Source: three-view drawing plus pictorial views. Frame: mm from the lowest corner of the part. Give positions to 0.01 mm unless a question says otherwise; leave off trailing zeros. Write each loop counter-clockwise with the first axis right and the second up, starting at its lowest first coordinate (ties: lowest second). Pieces come first, ordered by that corner, then holes.
Q1. Cut plane A-A on z = 32. Return the cut outline in (x, y).
Q2. Line query: L1, parallel to X at y = 2.05, z = 3.5; L2, parallel to X at y = 2.55, z = 32; L3, parallel to Z at x = 79.5, y = 2. Output: solid intervals per line, ascending.
Q3. Cut plane B-B on x = 79.5. Return the cut outline in (y, z), plus the area to 3 significant figures.
Q4. Cut plane C-C on z = 3.5. Return the cut outline in (x, y), plus the area to 3 significant figures.
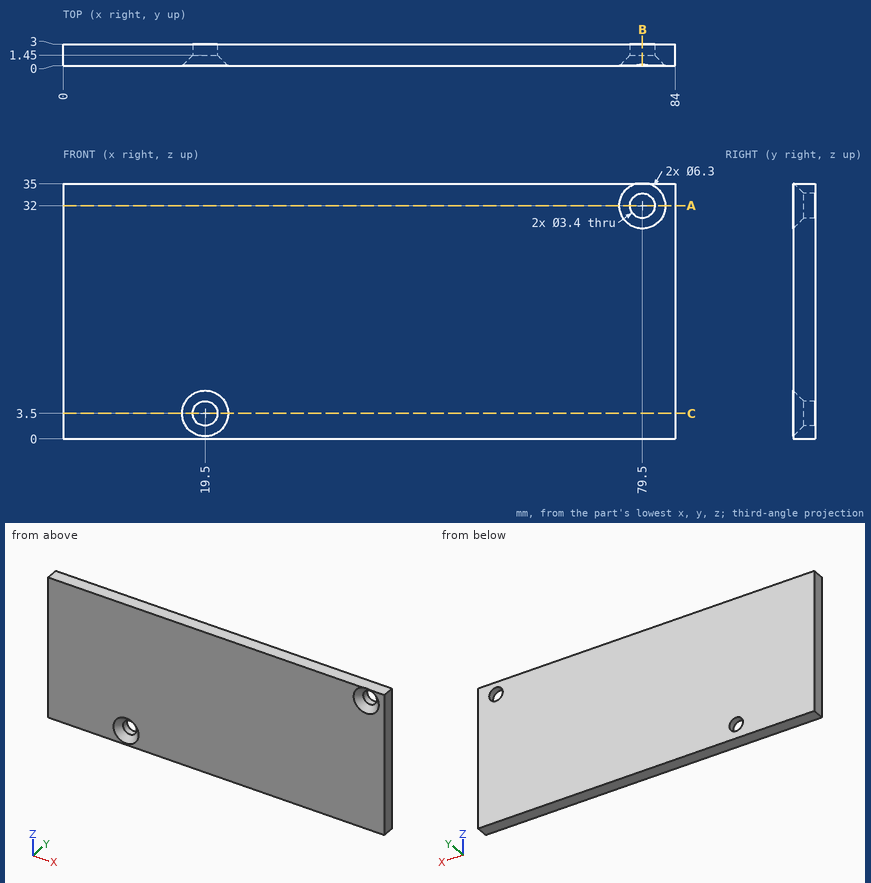
Data:
1. outline: (0, 0) - (76.35, 0) - (77.8, 1.45) - (77.8, 3) - (0, 3) - close; (81.2, 1.45) - (82.65, 0) - (84, 0) - (84, 3) - (81.2, 3) - close
2. L1: x = 0 to 17.8, 21.2 to 84
2. L2: x = 0 to 77.8, 81.2 to 84
2. L3: z = 0 to 30.3, 33.7 to 35
3. outline: (0, 0) - (3, 0) - (3, 30.3) - (1.45, 30.3) - (0, 28.85) - close; (0.15, 35) - (1.45, 33.7) - (3, 33.7) - (3, 35) - close
3. area: 92.7 mm2
4. outline: (0, 0) - (16.35, 0) - (17.8, 1.45) - (17.8, 3) - (0, 3) - close; (21.2, 1.45) - (22.65, 0) - (84, 0) - (84, 3) - (21.2, 3) - close
4. area: 240 mm2
